from build123d import *

# Parameters (mm, degrees)
F0_R     = 1
F0_R_2   = 4
F1_DEPTH = 8


# Not quite as in the source:
# - a feature names something its author has since deleted; it is built from what else it names


with BuildPart() as f1:
    # F0 (on Front) → F1 (new body)
    with BuildSketch(Plane.XZ):
        with BuildLine():
            Line((11, -17.5), (11, 17.5))
            ThreePointArc((11, 17.5), (0, 28.5), (-11, 17.5))
            Line((-11, 17.5), (-11, -17.5))
            Line((-11, -17.5), (-11, -28.5))
            Line((-11, -28.5), (0, -28.5))
            Line((0, -28.5), (11, -28.5))
            Line((11, -28.5), (11, -17.5))
        make_face()
        with Locations((0, -17.5)):
            Circle(F0_R, mode=Mode.SUBTRACT)
        Circle(F0_R_2, mode=Mode.SUBTRACT)
    extrude(amount=-F1_DEPTH)


solid = f1.part
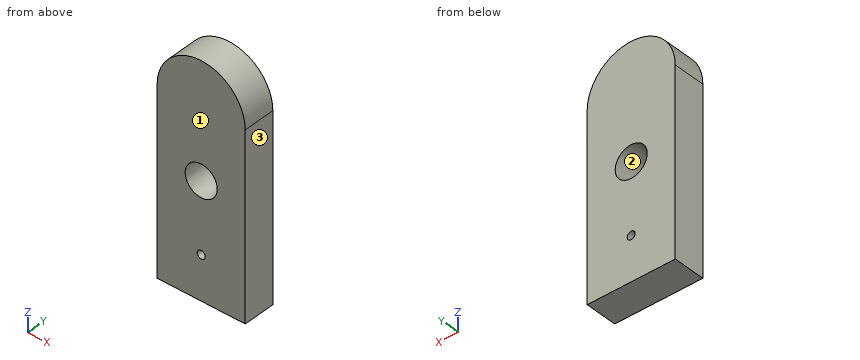
Verification items for the finished model (mm, model axes). Face numbers are marked on the shaded views. Give positions to 0.01 mm unless a question says otherwise; leave off trailing zeros. Write each loop counter-clockwise with the first axis right and the second up, starting at its lowest first coordinate (ties: lowest second). Pieces come first, ordered by that corner, then holes.
(1) Cross-section at A-A (x = 0). Enter the section's corners in (y, z), plus the area to 3 significant figures.
(2) Cross-section at B-B (z = 0). Enter the section's corners in (x, y).
(3) Cross-section at C-C (y = 1.5). Enter the section's corners in (x, z).
(4) Cross-section at D-D (z = -17.5). Enter the section's corners in (x, y), plus the area to 3 significant figures.
(5) Material ranges on line 1 (Z direction, x = 0, y = 5.75); line 2 (Z direction, x = 0.75, y = 5.25); line 3 (X direction, y = 7.75, z = 18), recorded low to high.
(6) Mould release check, pull along X, two halves, no side actions. Record for the marked faces 1, 2 and 3: +X half, -X half, draft (parallel to the pull), parting line (faces both ways), or undercut.
Worked out:
1. outline: (0, -28.5) - (8, -28.5) - (8, -18.5) - (0, -18.5) - close; (0, -16.5) - (8, -16.5) - (8, -4) - (0, -4) - close; (0, 4) - (8, 4) - (8, 28.5) - (0, 28.5) - close
1. area: 376 mm2
2. outline: (-11, 0) - (-4, 0) - (-4, 8) - (-11, 8) - close; (4, 0) - (11, 0) - (11, 8) - (4, 8) - close
3. outline: (-11, -28.5) - (11, -28.5) - (11, 17.5) arc R11 ccw to (-11, 17.5) - close; hole circle Ø8 at (0, 0); hole circle Ø2 at (0, -17.5)
4. outline: (-11, 0) - (-1, 0) - (-1, 8) - (-11, 8) - close; (1, 0) - (11, 0) - (11, 8) - (1, 8) - close
4. area: 160 mm2
5. line 1: z = -28.5 to -18.5, -16.5 to -4, 4 to 28.5
5. line 2: z = -28.5 to -18.16, -16.84 to -3.93, 3.93 to 28.47
5. line 3: x = -10.99 to 10.99
6. face 1: draft
6. face 2: undercut
6. face 3: +X half
